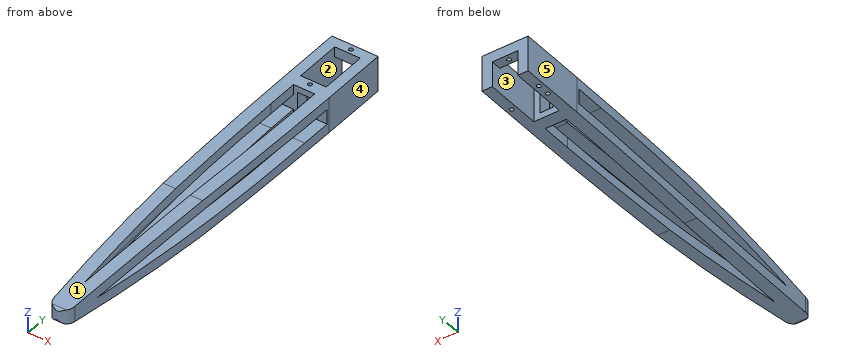
```python
from build123d import *

# Parameters (mm, degrees)
BOSS_EXTRUDE2_DEPTH      = 5
SKETCH4_W                = 12.4
SKETCH4_H                = 22.9
CUT_EXTRUDE1_DEPTH       = 5
SKETCH5_R                = 1
CUT_EXTRUDE2_DEPTH       = 5
CUT_EXTRUDE3_DEPTH       = 5
SKETCH6_W                = 5
SKETCH6_H                = 22.9
BOSS_EXTRUDE3_DEPTH      = 12.3
SKETCH7_R                = 1
CUT_EXTRUDE4_DEPTH       = 5
BOSS_EXTRUDE4_DEPTH      = 12.3
CUT_EXTRUDE5_DEPTH       = 121
CUT_EXTRUDE7_DEPTH       = 185.302285774
CUT_EXTRUDE8_DEPTH       = 121
CUT_EXTRUDE12_DEPTH      = 60.5
CUT_EXTRUDE13_REACH      = 174.902
SKETCH16_W               = 6.4
SKETCH16_H               = 11.3
CUT_EXTRUDE14_DEPTH      = 185.703363647
SKETCH23_W               = 7.3
SKETCH23_H               = 15
CUT_EXTRUDE15_DEPTH      = 185.687725676
CUT_EXTRUDE15_DEPTH_BACK = 185.687725676
SKETCH24_W               = 5
SKETCH24_H               = 12.3
BOSS_EXTRUDE5_DEPTH      = 5
BOSS_EXTRUDE6_REACH      = 187.32
SKETCH25_W               = 17.3
SKETCH25_H               = 5
BOSS_EXTRUDE7_REACH      = 187.32
SKETCH26_W               = 5
SKETCH26_H               = 5


with BuildPart() as part:
    # Sketch1 → Boss-Extrude2 (new body)
    with BuildSketch(Plane.XY):
        with BuildLine():
            Line((-6.2, 16.45), (6.2, 16.45))
            ThreePointArc((6.2, 16.45), (9.735533906, 14.985533906), (11.2, 11.45))
            Line((11.2, 11.45), (11.2, -16.45))
            ThreePointArc((11.2, -16.45), (9.649433537, -97.559262726), (5, -178.55))
            ThreePointArc((5, -178.55), (0, -183.55), (-5, -178.55))
            ThreePointArc((-5, -178.55), (-9.649433537, -97.559262726), (-11.2, -16.45))
            Line((-11.2, -16.45), (-11.2, 11.45))
            ThreePointArc((-11.2, 11.45), (-9.735533906, 14.985533906), (-6.2, 16.45))
        make_face()
    extrude(amount=BOSS_EXTRUDE2_DEPTH)

    # Sketch4 → Cut-Extrude1 (cut)
    with BuildSketch(Plane.XY.offset(5)):
        Rectangle(SKETCH4_W, SKETCH4_H)
    extrude(amount=-CUT_EXTRUDE1_DEPTH, mode=Mode.SUBTRACT)

    # Sketch5 → Cut-Extrude2 (cut)
    with BuildSketch(Plane.XY.offset(5)):
        with Locations((0, 13.8)):
            Circle(SKETCH5_R)
        with Locations((0, -13.8)):
            Circle(SKETCH5_R)
    extrude(amount=-CUT_EXTRUDE2_DEPTH, mode=Mode.SUBTRACT)

    # 3DSketch1 → Cut-Extrude3 (cut)
    with BuildSketch(Plane(origin=(-5.160423987, -32.686439405, 5), x_dir=(0.03897452460138957, -0.9992402045715013, 0), z_dir=(0, 0, 1))):
        with BuildLine():
            Line((0, 0), (0.402250143, 10.313006243))
            add(Edge.make_bspline(
                [(132.405052787, 0), (132.33638536, 0.007627552), (132.26771744, 0.015250757), (132.19904902, 0.022869576), (126.769998736, 0.624873123), (121.337777255, 1.198987474), (115.971798773, 1.743277878), (102.55225111, 3.059162741), (89.125108856, 4.291856269), (81.065896409, 4.997231834), (64.94123124, 6.330918517), (48.803313346, 7.493309622), (40.731510594, 8.035951572), (27.824174172, 8.848610973), (14.911969374, 9.58457196), (10.076236862, 9.846020434), (5.23968635, 10.089957993), (0.402250143, 10.313006243)],
                knots=[0, 0, 0, 0, 0, 0, 0.002323761, 0.002323761, 0.002323761, 0.183719441, 0.183719441, 0.183719441, 0.455812961, 0.455812961, 0.455812961, 0.72790648, 0.72790648, 0.72790648, 0.890780205, 0.890780205, 0.890780205, 0.890780205, 0.890780205, 0.890780205], degree=5))
            add(Edge.make_bspline(
                [(0, 0), (4.840113133, -0.15441643), (9.680970327, -0.287938029), (14.522375928, -0.403938196), (27.452676969, -0.675942436), (40.384098451, -0.871102077), (48.473645133, -0.958819983), (64.653074032, -1.056939836), (80.832632652, -0.983252259), (88.922302572, -0.907750283), (102.404667084, -0.724639456), (115.885939838, -0.457998492), (121.278011015, -0.333316775), (126.738446926, -0.184061374), (132.197893558, -0.0067545), (132.266946789, -0.004507398), (132.335999865, -0.002255886), (132.405052787, 0)],
                knots=[0.109219795, 0.109219795, 0.109219795, 0.109219795, 0.109219795, 0.109219795, 0.27209352, 0.27209352, 0.27209352, 0.544187039, 0.544187039, 0.544187039, 0.816280559, 0.816280559, 0.816280559, 0.997676239, 0.997676239, 0.997676239, 1, 1, 1, 1, 1, 1], degree=5))
        make_face()
    extrude(amount=-CUT_EXTRUDE3_DEPTH, mode=Mode.SUBTRACT)

    # Sketch6 → Boss-Extrude3 (add)
    with BuildSketch(Plane(origin=(0, 0, 0), x_dir=(-1, 0, 0), z_dir=(0, 0, -1))):
        with Locations((-8.7, 0)):
            Rectangle(SKETCH6_W, SKETCH6_H)
        with Locations((8.7, 0)):
            Rectangle(SKETCH6_W, SKETCH6_H)
    extrude(amount=BOSS_EXTRUDE3_DEPTH)

    # Sketch7 → Cut-Extrude4 (cut)
    with BuildSketch(Plane(origin=(0, 0, -12.3), x_dir=(-1, 0, 0), z_dir=(0, 0, -1))):
        with Locations((-8.665838134, 0)):
            Circle(SKETCH7_R)
        with Locations((8.880503913, 0)):
            Circle(SKETCH7_R)
        with Locations((8.880503913, 6)):
            Circle(SKETCH7_R)
    extrude(amount=-CUT_EXTRUDE4_DEPTH, mode=Mode.SUBTRACT)

    # Sketch8 → Boss-Extrude4 (add)
    with BuildSketch(Plane(origin=(0, 0, 0), x_dir=(-1, 0, 0), z_dir=(0, 0, -1))):
        with BuildLine():
            Line((11.2, -16.45), (11.2, -11.45))
            Line((11.2, -11.45), (6.2, -11.45))
            Line((6.2, -11.45), (-6.2, -11.45))
            Line((-6.2, -11.45), (-11.2, -11.45))
            Line((-11.2, -11.45), (-11.2, -16.45))
            ThreePointArc((-11.2, -16.45), (-9.649433537, -97.559262726), (-5, -178.55))
            ThreePointArc((-5, -178.55), (0, -183.55), (5, -178.55))
            ThreePointArc((5, -178.55), (9.649433537, -97.559262726), (11.2, -16.45))
        make_face()
    extrude(amount=BOSS_EXTRUDE4_DEPTH)

    # Sketch10 → Cut-Extrude5 (cut)
    with BuildSketch(Plane.XY):
        with BuildLine():
            Line((5.16042399, -32.686439405), (-5.160423987, -32.686439405))
            add(Edge.make_bspline(
                [(-5.160423987, -32.686439405), (-5.126081984, -37.528893349), (-5.070832025, -42.371276423), (-4.998052574, -47.213524597), (-4.765897811, -60.144602491), (-4.456913166, -73.073804992), (-4.229278188, -81.160624037), (-3.69673794, -97.331584054), (-2.992515745, -113.495977582), (-2.601780096, -121.576558353), (-1.893339649, -135.041542369), (-1.10147508, -148.502179909), (-0.766734685, -153.885294805), (-0.404774794, -159.335764743), (-0.0148233, -164.784152861), (-0.009886589, -164.853066046), (-0.004945476, -164.921978904), (1e-09, -164.990891438)],
                knots=[0.109219795, 0.109219795, 0.109219795, 0.109219795, 0.109219795, 0.109219795, 0.27209352, 0.27209352, 0.27209352, 0.544187039, 0.544187039, 0.544187039, 0.816280559, 0.816280559, 0.816280559, 0.997676239, 0.997676239, 0.997676239, 1, 1, 1, 1, 1, 1], degree=5))
            add(Edge.make_bspline(
                [(1e-09, -164.990891438), (0.004945477, -164.921978904), (0.00988659, -164.853066046), (0.014823301, -164.784152861), (0.404774795, -159.335764743), (0.766734686, -153.885294805), (1.101475081, -148.502179909), (1.89333965, -135.041542369), (2.601780097, -121.576558353), (2.992515747, -113.495977582), (3.696737942, -97.331584054), (4.22927819, -81.160624037), (4.456913168, -73.073804992), (4.765897813, -60.144602491), (4.998052577, -47.213524597), (5.070832028, -42.371276423), (5.126081987, -37.528893349), (5.16042399, -32.686439405)],
                knots=[0, 0, 0, 0, 0, 0, 0.002323761, 0.002323761, 0.002323761, 0.183719441, 0.183719441, 0.183719441, 0.455812961, 0.455812961, 0.455812961, 0.72790648, 0.72790648, 0.72790648, 0.890780205, 0.890780205, 0.890780205, 0.890780205, 0.890780205, 0.890780205], degree=5))
        make_face()
    extrude(amount=-CUT_EXTRUDE5_DEPTH, mode=Mode.SUBTRACT)

    # Sketch12 → Cut-Extrude7 (cut, through all)
    with BuildSketch(Plane(origin=(0, 0, 0), x_dir=(0, 0, -1), z_dir=(1, 0, 0))):
        with BuildLine():
            Line((0, -32.686439405), (7.3, -32.686439405))
            ThreePointArc((7.3, -32.686439405), (7.305216991, -98.889157238), (3.65, -164.99089144))
            ThreePointArc((3.65, -164.99089144), (-0.005216991, -98.889157238), (0, -32.686439405))
        make_face()
    extrude(amount=-CUT_EXTRUDE7_DEPTH, mode=Mode.SUBTRACT)

    # Sketch14 → Cut-Extrude8 (cut)
    with BuildSketch(Plane(origin=(0, 0, 0), x_dir=(0, 0, -1), z_dir=(1, 0, 0))):
        with BuildLine():
            Line((7.3, -32.686439405), (0, -32.686439405))
            ThreePointArc((0, -32.686439405), (-0.005216991, -98.889157238), (3.65, -164.99089144))
            ThreePointArc((3.65, -164.99089144), (7.305216991, -98.889157238), (7.3, -32.686439405))
        make_face()
    extrude(amount=CUT_EXTRUDE8_DEPTH, mode=Mode.SUBTRACT)

    # Sketch15 → Cut-Extrude12 (cut, symmetric)
    with BuildSketch(Plane(origin=(0, 0, 0), x_dir=(0, 0, -1), z_dir=(1, 0, 0))):
        with BuildLine():
            Line((12.301916168, -32.686439405), (24.156676666, -32.686439405))
            Line((24.156676666, -32.686439405), (24.156676666, -183.55))
            Line((24.156676666, -183.55), (5.626116445, -183.55))
            ThreePointArc((5.626116445, -183.55), (6.634148123, -183.160797973), (7.119075837, -182.195162848))
            ThreePointArc((7.119075837, -182.195162848), (12.038912499, -107.52151756), (12.301916168, -32.686439405))
        make_face()
        with BuildLine():
            Line((-5.001916168, -32.686439405), (-15.644111431, -32.686439405))
            Line((-15.644111431, -32.686439405), (-15.644111431, -183.55))
            Line((-15.644111431, -183.55), (1.673883555, -183.55))
            ThreePointArc((1.673883555, -183.55), (0.665851877, -183.160797973), (0.180924163, -182.195162848))
            ThreePointArc((0.180924163, -182.195162848), (-4.738912499, -107.52151756), (-5.001916168, -32.686439405))
        make_face()
    extrude(amount=CUT_EXTRUDE12_DEPTH, both=True, mode=Mode.SUBTRACT)

    # Sketch16 → Cut-Extrude13 (cut, up to next)
    with BuildSketch(Plane(origin=(0, -11.45, 0), x_dir=(1, 0, 0), z_dir=(0, 1, 0)), mode=Mode.PRIVATE) as cut_extrude13_sk1:
        with Locations((0, 3.65)):
            Rectangle(SKETCH16_W, SKETCH16_H)
    cut_extrude13_tool1 = extrude(cut_extrude13_sk1.sketch, amount=-CUT_EXTRUDE13_REACH, mode=Mode.PRIVATE) & part.part
    add(cut_extrude13_tool1.solids().sort_by_distance((0, -11.45, -3.65))[0], mode=Mode.SUBTRACT)

    # Sketch21 → Cut-Extrude14 (cut, through all)
    with BuildSketch(Plane.XY.offset(5)):
        Polygon((-5.160423987, -32.686439405), (5.16042399, -32.686439405), (5.160423987, -17.686439405), (-5.160423987, -17.686439405), align=None)
    extrude(amount=-CUT_EXTRUDE14_DEPTH, mode=Mode.SUBTRACT)

    # Sketch23 → Cut-Extrude15 (cut, two sides)
    with BuildSketch(Plane(origin=(-5.160423987, 0, 0), x_dir=(0, 0, -1), z_dir=(1, 0, 0))) as cut_extrude15_sk:
        with Locations((3.65, -25.186439405)):
            Rectangle(SKETCH23_W, SKETCH23_H)
    extrude(amount=CUT_EXTRUDE15_DEPTH, mode=Mode.SUBTRACT)
    extrude(cut_extrude15_sk.sketch, amount=-CUT_EXTRUDE15_DEPTH_BACK, mode=Mode.SUBTRACT)

    # Sketch24 → Boss-Extrude5 (add)
    with BuildSketch(Plane(origin=(0, 11.45, 0), x_dir=(1, 0, 0), z_dir=(0, 1, 0))):
        with Locations((8.7, 6.15)):
            Rectangle(SKETCH24_W, SKETCH24_H)
        with Locations((-8.7, 6.15)):
            Rectangle(SKETCH24_W, SKETCH24_H)
    extrude(amount=BOSS_EXTRUDE5_DEPTH)

    # Sketch25 → Boss-Extrude6 (add, up to next)
    with BuildSketch(Plane(origin=(11.2, 0, 0), x_dir=(0, 0, -1), z_dir=(1, 0, 0)), mode=Mode.PRIVATE) as boss_extrude6_sk1:
        with Locations((3.65, 13.95)):
            Rectangle(SKETCH25_W, SKETCH25_H)
    boss_extrude6_tool1 = extrude(boss_extrude6_sk1.sketch, amount=-BOSS_EXTRUDE6_REACH, mode=Mode.PRIVATE) - part.part
    add(boss_extrude6_tool1.solids().sort_by_distance((11.2, 13.95, -3.65))[0])

    # Sketch26 → Boss-Extrude7 (add, up to next)
    with BuildSketch(Plane.ZY.offset(11.2), mode=Mode.PRIVATE) as boss_extrude7_sk1:
        with Locations((2.5, 13.95)):
            Rectangle(SKETCH26_W, SKETCH26_H)
    boss_extrude7_tool1 = extrude(boss_extrude7_sk1.sketch, amount=-BOSS_EXTRUDE7_REACH, mode=Mode.PRIVATE) - part.part
    add(boss_extrude7_tool1.solids().sort_by_distance((-11.2, 13.95, 2.5))[0])


solid = part.part
```
Input: part model. Units: mm. Frame: model coordinates. Face numbers are marked on the shaded views. A direction names the side the tool comes from. Coordinates: 2 decimals unless noted, no trailing zeros. Order: outer loops, then holes, each group sorted by start corner. A loop starts at its lowest first (then second) coordinate and runs counter-clockwise, first axis right, second up. Notation, with made-up numbers: (85.5, -40) - (92.5, -40) arc R7 cw to (92.5, -29) - close; hole circle Ø6 at (76, 6.25). An arc over 180 degrees is marked (long way). Put each result on its own line as item: value.
1. Draft query along X for the marked faces 3, 4 and 5. Return one class per face: pulls with the +X half, pulls with the -X half, needs draft (parallel to the pull), parting line crosses it, or undercut.
Report:
face 3: undercut
face 4: pulls with the +X half
face 5: pulls with the -X half
2. Cut plane B-B on y = -136.5. State how many separate pieces and enclosed holes the cut face has, then the cut area to 3 significant figures.
Report:
separate pieces: 4
enclosed holes: 0
area: 120 mm2
3. Cut plane A-A on y = -29.5. Return the cut outline in (x, z), then the cut area to 3 significant figures.
Report:
outline: (-11.16, -12.3) - (-5.16, -12.3) - (-5.16, -7.3) - (-11.16, -7.3) - close; (-11.16, 0) - (-5.16, 0) - (-5.16, 5) - (-11.16, 5) - close; (5.16, -12.3) - (11.16, -12.3) - (11.16, -7.3) - (5.16, -7.3) - close; (5.16, 0) - (11.16, 0) - (11.16, 5) - (5.16, 5) - close
area: 120 mm2
4. Reachability of the marked faces 1 and 2 from +Z, -Z, +X, -X, +Y, -Y: full face, straight path, thin tool, end or side. Return the list, or none.
Report:
face 1: +Z, +X, -X, -Y
face 2: -Z
5. Contact query for flat-ended pins moving along their axis: pin 1 Ø4 at (y, z) = (-101, -7.5) entering from +X; pin 2 Ø3 at (x, z) = (4.5, -7) entering from +Y; pin 3 Ø4 at (y, z) = (-104, -7.5) entering from +X. Output: stop coordinate, or through.
Report:
pin 1: stops at x = 9.59
pin 2: stops at y = -11.45
pin 3: stops at x = 9.47
6. Line query: line 1 along Z through (x, y) = (-9.5, -62.5); line 2 along X through (y, z) = (-34, -10.5); line 3 along Y through (x, z) = (-9.5, -0.25). Output: solid intervals per line, ascending.
Report:
line 1: z = -12.3 to -7.76, 0.46 to 5
line 2: x = -11.13 to -5.15, 5.15 to 11.13
line 3: y = -17.69 to 16.45
